Can you work these out from the model? Positions are in its coordinate system, mm. Coordinates: 2 decimals unless noted, no trailing zeros. Order: outer loops, then holes, each group sorted by start corner. A loop starts at its lowest first (then second) coordinate and runs counter-clockwise, first axis right, second up. Notation, with made-up numbers: (-33, -35) - (26, -35) arc R26 ccw to (26, -4) - close; hole circle Ø3 at (-34.5, 51.25). An arc over 180 degrees is marked (long way). Return JSON: item names as keys, results as strings. Group by question number.
1) Imagine slicing it at A-A (y = -4). Write out the boundary of the cut face in (x, z), and give its area (3 significant figures).
2) Imagine slicing it at B-B (x = 22.5). Write out the boundary of the cut face in (y, z).
3) Imagine slicing it at C-C (x = 0). Write out the boundary of the cut face in (y, z), and give its area (3 significant figures).
4) If I drill on line 1 along Z through (x, y) = (24, -4.6); line 2 along Z through (x, y) = (0, -3.5); line 3 along X through (y, z) = (-0.2, 2.25), over which ranges is the centre line in solid material (lowest first)?
5) If we mould it in two halves opening along Z, with no side actions, what happens to faces 1 (the face through (25.955, -2.465, 1.325)), 2 (the face through (13, -2, -3.5)), 3 (the face through (12, 0, 0))? For each: pulls with the +Z half, pulls with the -Z half, needs draft (parallel to the pull), parting line crosses it, or undercut.
```python
from build123d import *

# Parameters (mm, degrees)
BLOCK_R                = 2.5
BOSS_EXTRUDE1_DEPTH    = 5
M3_TAPPED_HOLE1_D      = 2.5
M2_TAPPED_HOLE1_REACH  = 27.251
M2_TAPPED_HOLE1_BORE_R = 0.8


with BuildPart() as part:
    # block → Boss-Extrude1 (new body)
    with BuildSketch(Plane(origin=(0, 0, 0), x_dir=(1, 0, 0), z_dir=(0, 1, 0))):
        Polygon((0.732050808, 3.5), (25, 3.5), (27, 1.5), (27, -1.5), (25, -3.5), (0.732050808, -3.5), (-3, -2.5), (-3, 2.5), align=None)
        with Locations(Location((22.5, 0, 0), (0, 0, 270))):
            Circle(BLOCK_R, mode=Mode.SUBTRACT)
    extrude(amount=-BOSS_EXTRUDE1_DEPTH)

    # M3 Tapped Hole1 (through all)
    with Locations(Plane(origin=(0, 0, 0), x_dir=(1, 0, 0), z_dir=(0, 1, 0))):
        with Locations((0, 0)):
            Hole(M3_TAPPED_HOLE1_D / 2)

    # M2 Tapped Hole1 bore → M2 Tapped Hole1 (cut, up to next)
    with BuildSketch(Plane(origin=(14.25, 0, -14.25), x_dir=(-0.7071067811865465, 0, -0.7071067811865486), z_dir=(0.7071067811865486, 0, -0.7071067811865465)), mode=Mode.PRIVATE) as m2_tapped_hole1_sk1:
        with Locations((-16.617009358, -2.5)):
            Circle(M2_TAPPED_HOLE1_BORE_R)
    m2_tapped_hole1_tool1 = extrude(m2_tapped_hole1_sk1.sketch, amount=-M2_TAPPED_HOLE1_REACH, mode=Mode.PRIVATE) & part.part
    m2_tapped_hole1 = m2_tapped_hole1_tool1.solids().sort_by_distance((26, -2.5, -2.5))[0]
    add(m2_tapped_hole1, mode=Mode.SUBTRACT)

    # Mirror1: M2 Tapped Hole1 across plane
    add(m2_tapped_hole1.mirror(Plane.XY), mode=Mode.SUBTRACT)


solid = part.part
```
Calculated:
{
 "1": {"outline": "(-3, -2.5) - (0.73, -3.5) - (25, -3.5) - (27, -1.5) - (27, 1.5) - (25, 3.5) - (0.73, 3.5) - (-3, 2.5) - close; hole circle Ø2.5 at (0, 0); hole circle Ø5 at (22.5, 0)", "area": "178 mm2"},
 "2": {"outline": "(-5, -3.5) - (0, -3.5) - (0, -2.5) - (-5, -2.5) - close; (-5, 2.5) - (0, 2.5) - (0, 3.5) - (-5, 3.5) - close"},
 "3": {"outline": "(-5, -3.3) - (0, -3.3) - (0, -1.25) - (-5, -1.25) - close; (-5, 1.25) - (0, 1.25) - (0, 3.3) - (-5, 3.3) - close", "area": "20.5 mm2"},
 "4": {"line 1": "-3.5 to -2, 2 to 3.5", "line 2": "-3.3 to -1.25, 1.25 to 3.3", "line 3": "-3 to 21.41, 23.59 to 26.25"},
 "5": {"face 1": "undercut", "face 2": "pulls with the -Z half", "face 3": "needs draft"}
}
